Design review of the part built by this model. Coordinates are the model's own, in mm. A direction names the side the tool comes from. Give positions to 0.01 mm unless a question says otherwise; leave off trailing zeros. Write each loop counter-clockwise with the first axis right and the second up, starting at its lowest first coordinate (ties: lowest second). Pieces come first, ordered by that corner, then holes.
```python
from build123d import *
from OCP.BRepFilletAPI import BRepFilletAPI_MakeChamfer

# Parameters (mm, degrees)
ESQUISSE2_R        = 6.75
ESQUISSE2_R_2      = 158
BOSS_EXTRU_1_DEPTH = 10
BOSS_EXTRU_2_DEPTH = 10
CONG_1_R           = 15
CHANFREIN1_SIZE    = 140
CHANFREIN1_SIZE2   = 99.577969333
CHANFREIN1_SIZE2_2 = 103.340011173
CONG_2_R           = 10


with BuildPart() as part:
    # Esquisse2 → Boss.-Extru.1 (new body)
    with BuildSketch(Plane(origin=(0, 0, 0), x_dir=(1, 0, 0), z_dir=(0, 1, 0))):
        with BuildLine():
            Line((0, 0), (0, 525))
            Line((0, 525), (-250, 1230.600775194))
            Line((-250, 1230.600775194), (330.895152108, 704.538780798))
            ThreePointArc((330.895152108, 704.538780798), (394.393669115, 575.365591696), (351.977546011, 437.820519282))
            Line((351.977546011, 437.820519282), (0, 0))
        make_face()
        with Locations(Location((200, 380, 0), (0, 0, 270))):
            Circle(ESQUISSE2_R, mode=Mode.SUBTRACT)
        with Locations(Location((144.376941013, 388.809827067, 0), (0, 0, 270))):
            Circle(ESQUISSE2_R, mode=Mode.SUBTRACT)
        with Locations(Location((94.198654587, 414.376941013, 0), (0, 0, 270))):
            Circle(ESQUISSE2_R, mode=Mode.SUBTRACT)
        with Locations(Location((54.376941013, 454.198654587, 0), (0, 0, 270))):
            Circle(ESQUISSE2_R, mode=Mode.SUBTRACT)
        with Locations(Location((28.809827067, 504.376941013, 0), (0, 0, 270))):
            Circle(ESQUISSE2_R, mode=Mode.SUBTRACT)
        with Locations(Location((20, 560, 0), (0, 0, 270))):
            Circle(ESQUISSE2_R, mode=Mode.SUBTRACT)
        with Locations(Location((28.809827067, 615.623058987, 0), (0, 0, 270))):
            Circle(ESQUISSE2_R, mode=Mode.SUBTRACT)
        with Locations(Location((54.376941013, 665.801345413, 0), (0, 0, 270))):
            Circle(ESQUISSE2_R, mode=Mode.SUBTRACT)
        with Locations(Location((94.198654587, 705.623058987, 0), (0, 0, 270))):
            Circle(ESQUISSE2_R, mode=Mode.SUBTRACT)
        with Locations(Location((144.376941013, 731.190172933, 0), (0, 0, 270))):
            Circle(ESQUISSE2_R, mode=Mode.SUBTRACT)
        with Locations(Location((200, 740, 0), (0, 0, 270))):
            Circle(ESQUISSE2_R, mode=Mode.SUBTRACT)
        with Locations(Location((255.623058987, 731.190172933, 0), (0, 0, 270))):
            Circle(ESQUISSE2_R, mode=Mode.SUBTRACT)
        with Locations(Location((305.801345413, 705.623058987, 0), (0, 0, 270))):
            Circle(ESQUISSE2_R, mode=Mode.SUBTRACT)
        with Locations(Location((345.623058987, 665.801345413, 0), (0, 0, 270))):
            Circle(ESQUISSE2_R, mode=Mode.SUBTRACT)
        with Locations(Location((371.190172933, 615.623058987, 0), (0, 0, 270))):
            Circle(ESQUISSE2_R, mode=Mode.SUBTRACT)
        with Locations(Location((380, 560, 0), (0, 0, 270))):
            Circle(ESQUISSE2_R, mode=Mode.SUBTRACT)
        with Locations(Location((371.190172933, 504.376941013, 0), (0, 0, 270))):
            Circle(ESQUISSE2_R, mode=Mode.SUBTRACT)
        with Locations(Location((345.623058987, 454.198654587, 0), (0, 0, 270))):
            Circle(ESQUISSE2_R, mode=Mode.SUBTRACT)
        with Locations(Location((305.801345413, 414.376941013, 0), (0, 0, 270))):
            Circle(ESQUISSE2_R, mode=Mode.SUBTRACT)
        with Locations(Location((255.623058987, 388.809827067, 0), (0, 0, 270))):
            Circle(ESQUISSE2_R, mode=Mode.SUBTRACT)
        with Locations(Location((200, 560, 0), (0, 0, 270))):
            Circle(ESQUISSE2_R_2, mode=Mode.SUBTRACT)
        with BuildLine():
            Line((40, 113.596012676), (40, 411.932447849))
            ThreePointArc((40, 411.932447849), (124.193302514, 355.604930059), (224.754658533, 343.410048984))
            Line((224.754658533, 343.410048984), (40, 113.596012676))
        make_face(mode=Mode.SUBTRACT)
        with BuildLine():
            Line((190.419715338, 777.789389424), (-159.36047406, 1094.552342888))
            Line((-159.36047406, 1094.552342888), (-0.382744379, 645.853105682))
            ThreePointArc((-0.382744379, 645.853105682), (76.012443637, 739.307238747), (190.419715338, 777.789389424))
        make_face(mode=Mode.SUBTRACT)
    extrude(amount=BOSS_EXTRU_1_DEPTH)

    # Esquisse4 → Boss.-Extru.2 (add)
    with BuildSketch(Plane(origin=(0, 10, 0), x_dir=(1, 0, 0), z_dir=(0, 1, 0))):
        Polygon((349.666295471, 435), (400, 435), (400, 535), (393.390796058, 535), align=None)
    extrude(amount=-BOSS_EXTRU_2_DEPTH)

    # Congé1
    # the kernel refuses this fillet: 15 mm, written as the material it adds along each edge
    with BuildSketch(Plane(origin=(40, 0, -113.596012676), x_dir=(0, 0, -1), z_dir=(0, 1, 0))) as cong_1_piece_1:
        with BuildLine():
            CenterArc((CONG_1_R * 2.83990031691, -CONG_1_R), CONG_1_R, 90, 141.203115043)
            Line((CONG_1_R * 2.21333887733, -CONG_1_R * 1.77937203082), (0, 0))
            Line((0, 0), (CONG_1_R * 2.83990031691, 0))
        make_face()
    extrude(amount=10)
    with BuildSketch(Plane(origin=(224.754658533, 0, -343.410048984), x_dir=(-0.9991751199955, 0, 0.040608860880086604), z_dir=(0, 1, 0))) as cong_1_piece_2:
        with BuildLine():
            CenterArc((32.974239643, 14.959854274), CONG_1_R, 138.875758739, 126.931398571)
            Line((21.674961702, 24.825264453), (0, 0))
            ThreePointArc((0, 0), (15.938767721, 0.58345122), (31.877535442, 0))
        make_face()
    extrude(amount=10)
    with BuildSketch(Plane(origin=(40, 0, -411.932447849), x_dir=(0.7331146005810171, 0, 0.6801051260025437), z_dir=(0, 1, 0))) as cong_1_piece_3:
        with BuildLine():
            CenterArc((34.335653812, -14.956465907), CONG_1_R, 94.366282627, 128.48557588)
            Line((23.338934803, -25.158042797), (0, 0))
            ThreePointArc((0, 0), (16.59683488, -0.632695485), (33.193669761, 0))
        make_face()
    extrude(amount=10)
    with BuildSketch(Plane(origin=(-0.382744379, 0, -645.853105682), x_dir=(0.4627745806888944, 0, -0.8864759937348659), z_dir=(0, 1, 0))) as cong_1_piece_4:
        with BuildLine():
            CenterArc((34.394590931, 14.956316108), CONG_1_R, 137.075935051, 128.550273023)
            Line((23.410737088, 25.1717434), (0, 0))
            ThreePointArc((0, 0), (16.625323332, 0.634872567), (33.250646665, 0))
        make_face()
    extrude(amount=10)
    with BuildSketch(Plane(origin=(190.419715338, 0, -777.789389424), x_dir=(-0.9931470305035408, 0, 0.11687162102922555), z_dir=(0, 1, 0))) as cong_1_piece_5:
        with BuildLine():
            CenterArc((32.974239643, -14.959854274), CONG_1_R, 94.19284269, 126.931398571)
            Line((21.674961702, -24.825264453), (0, 0))
            ThreePointArc((0, 0), (15.938767721, -0.58345122), (31.877535442, 0))
        make_face()
    extrude(amount=10)
    with BuildSketch(Plane(origin=(-159.36047406, 0, -1094.552342888), x_dir=(0.3339655112300271, 0, 0.942585294447599), z_dir=(0, 1, 0))) as cong_1_piece_6:
        with BuildLine():
            CenterArc((CONG_1_R * 3.96269318106, CONG_1_R), CONG_1_R, 118.326186848, 151.673813152)
            Line((CONG_1_R * 3.48820260226, CONG_1_R * 1.88026058109), (0, 0))
            Line((0, 0), (CONG_1_R * 3.96269318106, 0))
        make_face()
    extrude(amount=10)
    with BuildSketch(Plane(origin=(393.390796058, 10, -535), x_dir=(1, 0, 0), z_dir=(0, -1, 0))) as cong_1_piece_7:
        with BuildLine():
            CenterArc((16.178133023, -11.551432649), CONG_1_R, 129.637533665, 54.034246436)
            ThreePointArc((1.208923803, -12.512044602), (0.705308812, -6.246278392), (0, 0))
            Line((0, 0), (6.609203942, 0))
        make_face()
    extrude(amount=10)
    with BuildSketch(Plane(origin=(349.71004275, 10, -435), x_dir=(1, 0, 0), z_dir=(0, -1, 0))) as cong_1_piece_8:
        with BuildLine():
            CenterArc((CONG_1_R * 0.479153145931, CONG_1_R), CONG_1_R, 218.796884957, 51.203115043)
            Line((-CONG_1_R * 0.300218884894, CONG_1_R * 0.37343856042), (0, 0))
            Line((0, 0), (CONG_1_R * 0.479153145931, 0))
        make_face()
    extrude(amount=10)
    # the kernel refuses this fillet: 15 mm, written as the material it takes off along each edge
    with BuildSketch(Plane(origin=(400, 47.5, -435), x_dir=(0, 0, -1), z_dir=(0, -1, 0))) as cong_1_2_piece_1:
        with BuildLine():
            CenterArc((CONG_1_R, -CONG_1_R), CONG_1_R, 90, 90)
            Line((0, -CONG_1_R), (0, 0))
            Line((0, 0), (CONG_1_R, 0))
        make_face()
    extrude(amount=85, mode=Mode.SUBTRACT)

    # Chanfrein1: one chamfer whose edges measure the first distance from different faces: ONE call of the kernel's chamfer builder (chamfer() names one face for all edges)
    chanfrein1_edges_1 = [part.edges().sort_by_distance(p)[0] for p in [
        (0, 5, 0),
    ]]
    chanfrein1_side_1 = [part.faces().sort_by_distance(p)[0] for p in [
        (172.603379738, 5, -214.699210797),
    ]]
    chanfrein1_edges_2 = [part.edges().sort_by_distance(p)[0] for p in [
        (-250, 5, -1230.600775194),
    ]]
    chanfrein1_side_2 = [part.faces().sort_by_distance(p)[0] for p in [
        (40.447576054, 5, -967.569777996),
    ]]
    chanfrein1 = BRepFilletAPI_MakeChamfer(part.part.solid().wrapped)
    for e in chanfrein1_edges_1:
        chanfrein1.Add(CHANFREIN1_SIZE, CHANFREIN1_SIZE2, e.wrapped, chanfrein1_side_1[0].wrapped)  # the first distance lies on this face
    for e in chanfrein1_edges_2:
        chanfrein1.Add(CHANFREIN1_SIZE, CHANFREIN1_SIZE2_2, e.wrapped, chanfrein1_side_2[0].wrapped)  # the first distance lies on this face
    add(Compound.cast(chanfrein1.Shape()), mode=Mode.REPLACE)

    # Congé2
    cong_2_edges = [part.edges().sort_by_distance(p)[0] for p in [
        (400, 5, -535),
    ]]
    fillet(cong_2_edges, radius=CONG_2_R)


solid = part.part
```
(1) Consider section A-A, the plane x = -77. Give the boundary of the cut face in (y, z), then the cut area to 3 significant figures.
Resolved:
outline: (0, -1073.93) - (10, -1073.93) - (10, -1019.97) - (0, -1019.97) - close; (0, -862.1) - (10, -862.1) - (10, -742.33) - (0, -742.33) - close
area: 1,740 mm2
(2) Mouldability with a two-part tool opening along X and no side actions: class faces 3 (the face through (103.859, 4.93, -685.383)), 4 (the face through (-106.236, 4.93, -824.84)), 5 (the face through (218.265, 4.93, -271.497)), 6 (the face through (48, 0, -654)) as pulls with the +X half, pulls with the -X half, needs draft (parallel to the pull), parting line crosses it, or undercut.
Resolved:
face 3: undercut
face 4: pulls with the -X half
face 5: pulls with the +X half
face 6: needs draft
(3) Tool access review of faces 1 (the face through (-76.58, 4.93, -860.91)), 2 (the face through (48, 10, -654)): name each direction out of +Z, -Z, +X, -X, +Y, -Y from which nothing blocks a thin tool from reaching the whole face with its end or side.
Resolved:
face 1: +Y, -Y
face 2: +Z, -Z, +X, -X, +Y
(4) Consider section B-B, the plane x = 224. Give the boundary of the cut face in (y, z).
Resolved:
outline: (0, -801.34) - (10, -801.34) - (10, -716.17) - (0, -716.17) - close; (0, -403.83) - (10, -403.83) - (10, -278.63) - (0, -278.63) - close
(5) Consider section C-C, the plane y = 2.25. Give the number of separate pieces and of enclosed holes in the cut face, then the cut area to 3 significant figures.
Resolved:
separate pieces: 1
enclosed holes: 23
area: 130,000 mm2
(6) Clearance check with flat-ended pins moving along their axes: P1, Ø6, axis at x = -117.5, y = 3.5, coming from the -Z side; P2, Ø2, axis at y = 2.5, z = -245, coming from the +X side; P3, Ø5, axis at x = 375.5, y = 6, coming from the +Z side. State where each tip first meets the part, or that it passes through.
Resolved:
P1: stops at z = -1113.32
P2: stops at x = 197.77
P3: stops at z = -435
(7) To check wall thickness, follow L1, parallel to Z at x = 156.5, y = 9; L2, parallel to X at y = 6, z = -377.5; L3, parallel to Z at x = 189.5, y = 6. State the ranges of each line that lie inside material, in increasing order.
Resolved:
L1: z = -862.47 to -808.51, -773.62 to -711.89, -408.11 to -346.38, -258.51 to -194.67
L2: x = 0 to 40, 80.76 to 193.73, 206.27 to 303.48
L3: z = -832.59 to -717.65, -402.35 to -342.25, -299.56 to -235.72
